Input: part model. Units: mm. Frame: model coordinates. Round coordinates to 2 decimals unless told otherwise and drop trailing zeros. Loops run counter-clockwise (first coordinate to the right, second up) from the corner with the lowest first, then second, coordinate; pieces in that order, holes last.
1) Section B-B, the plane z = -9.5. Return loops of the section in (x, y).
2) Section A-A, the plane y = 1.75. Return loops of the section in (x, z) (3 decimals), and give its area (3 significant figures).
3) Section C-C, the plane z = -41.5. Return loops of the section in (x, y), and give its area (3 significant figures).
4) Ray query, line 1 along X through (y, z) = (0.1, -9); line 2 along Z through (x, y) = (-20.5, 1.65). Return the intervals inside material, ascending.
5) Section D-D, the plane x = -76.5. Return loops of the section in (y, z), and give its area (3 significant figures).
6) First-contact query: pin 1 (5.5 mm diameter, centred on x = -9.525, z = -92.075, fed in from -Y); pin 2 (1.1 mm diameter, centred on y = 1.5, z = -52, fed in from -X). Flat tips, straight axial feed; report the tip coordinate or a pass-through.
Autodesk Inventor part; units mm, degrees
ref_plane "YZ Plane" through (0, 0, 0) normal (1, 0, 0) x (0, 1, 0)
ref_plane "XZ Plane" through (0, 0, 0) normal (0, 1, 0) x (-1, 0, 0)
ref_plane "XY Plane" through (0, 0, 0) normal (0, 0, 1) x (1, 0, 0)
sketch "Sketch1" plane through (0, 0, 0) normal (0, 1, 0) x (-1, 0, 0)
  line L0 (0, 0) -> (101.6, 0)
  line L1 (101.6, 0) -> (101.6, -19.05)
  line L2 (101.6, -19.05) -> (0, -19.05)
  line L3 (0, -19.05) -> (0, 0)
  line L4 (0, 0) -> (19.05, 0)
  line L5 (19.05, 0) -> (19.05, -101.6)
  line L6 (19.05, -101.6) -> (0, -101.6)
  line L7 (0, -101.6) -> (0, 0)
  dimension "d0" = 101.6
  dimension "d1" = 19.05
  dimension "d2" = 19.05
  dimension "d3" = 101.6
extrude "Extrusion1" add sketch "Sketch1" along normal blind 2.286
sketch "Sketch2" plane through (0, 2.286, 0) normal (0, 1, 0) x (1, 0, 0)
  line L0 (0, 0) -> (0, 101.6)
  line L1 (-101.6, 0) -> (0, 0)
  point P0 (-34.925, 9.525)
  point P1 (-92.075, 9.525)
  point P2 (-9.525, 34.925)
  point P3 (-9.525, 92.075)
  dimension "d8" = 9.525
  dimension "d11" = 9.525
  dimension "d13" = 9.525
  dimension "d14" = 9.525
  dimension "d23" = 34.925
  dimension "d24" = 92.075
  dimension "d25" = 34.925
  dimension "d26" = 92.075
hole "Hole1" at (-34.925, 2.286, -9.525) at (-92.075, 2.286, -9.525) at (-9.525, 2.286, -34.925) at (-9.525, 2.286, -92.075) direction (0, -1, 0) diameter 6.35 end through all
properties part number "wood gusset" material "Steel, Alloy"
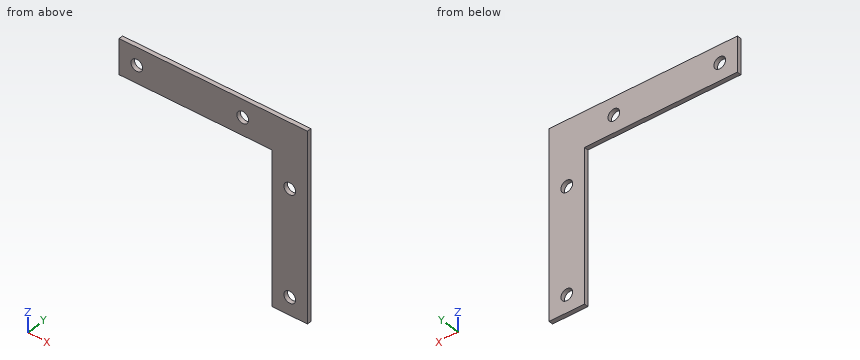
Final values:
1. outline: (-101.6, 0) - (-95.25, 0) - (-95.25, 2.29) - (-101.6, 2.29) - close; (-88.9, 0) - (-38.1, 0) - (-38.1, 2.29) - (-88.9, 2.29) - close; (-31.75, 0) - (0, 0) - (0, 2.29) - (-31.75, 2.29) - close
2. outline: (-101.6, -19.05) - (-19.05, -19.05) - (-19.05, -101.6) - (0, -101.6) - (0, 0) - (-101.6, 0) - close; hole circle Ø6.35 at (-92.075, -9.525); hole circle Ø6.35 at (-34.925, -9.525); hole circle Ø6.35 at (-9.525, -92.075); hole circle Ø6.35 at (-9.525, -34.925)
2. area: 3,380 mm2
3. outline: (-19.05, 0) - (0, 0) - (0, 2.29) - (-19.05, 2.29) - close
3. area: 43.5 mm2
4. line 1: x = -101.6 to -95.21, -88.94 to -38.06, -31.79 to 0
4. line 2: z = -19.05 to 0
5. outline: (0, -19.05) - (2.29, -19.05) - (2.29, 0) - (0, 0) - close
5. area: 43.5 mm2
6. pin 1: passes through
6. pin 2: stops at x = -19.05
